Geometry: final body of the model. Coordinates: model frame, mm. Face numbers are marked on the shaded views. A direction names the side the tool comes from. Coordinates: 2 decimals unless noted, no trailing zeros. Loops run counter-clockwise (first coordinate to the right, second up) from the corner with the lowest first, then second, coordinate; pieces in that order, holes last. Notation, with made-up numbers: (28, 54.25) - (78, 54.25) arc R16 cw to (78, 60.25) - close; hole circle Ø9 at (25, 72.25). An arc over 180 degrees is marked (long way). Put each result on its own line as item: value. Start each with the question number.
1) Section D-D on y = 10. Output: boundary loops of the cut face in (x, z).
2) Section C-C on z = 11. Output: boundary loops of the cut face in (x, y).
3) Reachability of the marked faces 1, 2 and 3 from +Z, -Z, +X, -X, +Y, -Y: full face, straight path, thin tool, end or side. Return the list, or none.
4) Section A-A on x = 7. Output: boundary loops of the cut face in (y, z).
5) Section B-B on y = 25. Output: boundary loops of the cut face in (x, z).
6) Material intervals for line 1 along Y through (x, z) = (5.75, 14.75); line 2 along Z through (x, y) = (7.5, 3); line 3 along X through (y, z) = (15, 11), sorted ascending. Write a range as from..to.
7) Contact query for flat-ended pins moving along their axis: pin 1 Ø3 at (x, z) = (4, 21) entering from -Y; pin 2 Ø5 at (y, z) = (19.5, 10) entering from +X; pin 3 Ø6.5 at (x, z) = (9, 10) entering from -Y. Output: stop coordinate, or through.
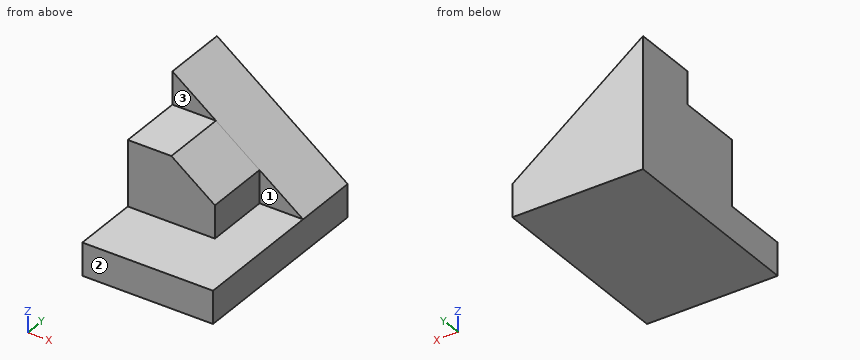
```python
from build123d import *

# Parameters (mm, degrees)
F0_W     = 25.4
F0_H     = 6.35
F1_DEPTH = 38.354
F3_DEPTH = 12.7
F5_DEPTH = 12.7
F6_DEPTH = 12.7


with BuildPart() as f1:
    # F0 (on Front) → F1 (new body)
    with BuildSketch(Plane.XZ):
        with Locations((12.7, 3.175)):
            Rectangle(F0_W, F0_H)
    extrude(amount=-F1_DEPTH)

    # F2 (on face) → F3 (join)
    with BuildSketch(Plane(origin=(0, 38.354, 0), x_dir=(-1, 0, 0), z_dir=(0, 1, 0))):
        Polygon((-25.4, 6.35), (0, 6.35), (0, 25.4), align=None)
    extrude(amount=-F3_DEPTH)

    # F4 (on face) → F5 (join)
    with BuildSketch(Plane.XZ.offset(-25.654)):
        Polygon((0, 6.35), (16.9333333333, 6.35), (16.9333333333, 12.7), (8.4666666667, 19.05), (0, 19.05), align=None)
    extrude(amount=F5_DEPTH)

    # F4 (on face) → F6 (join)
    with BuildSketch(Plane.XZ.offset(-25.654)):
        Polygon((0, 6.35), (16.9333333333, 6.35), (16.9333333333, 12.7), (8.4666666667, 19.05), (0, 19.05), align=None)
    extrude(amount=F6_DEPTH)


solid = f1.part
```
Answer block:
1. outline: (0, 0) - (25.4, 0) - (25.4, 6.35) - (0, 6.35) - close
2. outline: (0, 12.95) - (16.93, 12.95) - (16.93, 25.65) - (19.2, 25.65) - (19.2, 38.35) - (0, 38.35) - close
3. face 1: +Z, +X, -Y
3. face 2: +Z, -Z, +X, -X, -Y
3. face 3: +Z, +X, -X, -Y
4. outline: (0, 0) - (38.35, 0) - (38.35, 20.15) - (25.65, 20.15) - (25.65, 19.05) - (12.95, 19.05) - (12.95, 6.35) - (0, 6.35) - close
5. outline: (0, 0) - (25.4, 0) - (25.4, 6.35) - (16.93, 6.35) - (16.93, 12.7) - (8.47, 19.05) - (0, 19.05) - close
6. line 1: y = 12.95..38.35
6. line 2: z = 0..6.35
6. line 3: x = 0..16.93
7. pin 1: stops at y = 25.65
7. pin 2: stops at x = 16.93
7. pin 3: stops at y = 12.95
